Here's how the part is built. I have some questions about the finished solid (model axes, mm). Round coordinates to 2 decimals unless told otherwise and drop trailing zeros. Order: outer loops, then holes, each group sorted by start corner. A loop starts at its lowest first (then second) coordinate and runs counter-clockwise, first axis right, second up. Notation, with made-up numbers: (73, 21.25) - (78, 21.25) arc R28 cw to (78, 54.25) - close; hole circle Ø8 at (15.25, -1). An arc over 180 degrees is marked (long way). Answer as a JSON object with one key per item and string values.
```python
from build123d import *

# Parameters (mm, degrees)
SKETCH1_W           = 12.7
SKETCH1_H           = 25.4
SKETCH1_W_2         = 9.525
SKETCH1_H_2         = 22.225
BOSS_EXTRUDE1_DEPTH = 609.6
SKETCH2_R           = 3.81
SKETCH2_R_2         = 2.75
CUT_EXTRUDE1_DEPTH  = 610.86452594
CUT_EXTRUDE3_REACH  = 611.865
CUT_EXTRUDE5_REACH  = 612.162
SKETCH5_R           = 2.75


with BuildPart() as part:
    # Sketch1 → Boss-Extrude1 (new body)
    with BuildSketch(Plane.XY):
        Rectangle(SKETCH1_W, SKETCH1_H)
        Rectangle(SKETCH1_W_2, SKETCH1_H_2, mode=Mode.SUBTRACT)
    extrude(amount=BOSS_EXTRUDE1_DEPTH)

    # Sketch2 → Cut-Extrude1 (cut, through all)
    with BuildSketch(Plane(origin=(6.35, 0, 0), x_dir=(0, 0, -1), z_dir=(1, 0, 0))):
        with Locations((-571.5, 0)):
            Circle(SKETCH2_R)
        with Locations((-586.74, 0)):
            Circle(SKETCH2_R_2)
        with Locations((-556.26, 0)):
            Circle(SKETCH2_R_2)
        with Locations((-66.04, 0)):
            Circle(SKETCH2_R_2)
        with Locations((-35.56, 0)):
            Circle(SKETCH2_R_2)
        with Locations((-382.778, 0)):
            Circle(SKETCH2_R_2)
        with Locations((-398.018, 0)):
            Circle(SKETCH2_R)
        with Locations((-413.258, 0)):
            Circle(SKETCH2_R_2)
        with Locations((-209.296, 0)):
            Circle(SKETCH2_R_2)
        with Locations((-224.536, 0)):
            Circle(SKETCH2_R)
        with Locations((-239.776, 0)):
            Circle(SKETCH2_R_2)
        with BuildLine():
            Line((-44.45, -3.302), (-57.15, -3.302))
            ThreePointArc((-57.15, -3.302), (-60.452, 0), (-57.15, 3.302))
            Line((-57.15, 3.302), (-44.45, 3.302))
            ThreePointArc((-44.45, 3.302), (-41.148, 0), (-44.45, -3.302))
        make_face()
    extrude(amount=-CUT_EXTRUDE1_DEPTH, mode=Mode.SUBTRACT)

    # Sketch4 → Cut-Extrude3 (cut, up to next)
    with BuildSketch(Plane.ZY.offset(6.35), mode=Mode.PRIVATE) as cut_extrude3_sk1:
        with BuildLine():
            Line((35.56, 5), (66.04, 5))
            ThreePointArc((66.04, 5), (71.04, 0), (66.04, -5))
            Line((66.04, -5), (35.56, -5))
            ThreePointArc((35.56, -5), (30.56, 0), (35.56, 5))
        make_face()
    cut_extrude3_tool1 = extrude(cut_extrude3_sk1.sketch, amount=-CUT_EXTRUDE3_REACH, mode=Mode.PRIVATE) & part.part
    # Sketch4 → Cut-Extrude3 (cut, up to next)
    with BuildSketch(Plane.ZY.offset(6.35), mode=Mode.PRIVATE) as cut_extrude3_sk2:
        with BuildLine():
            Line((556.26, 5), (586.74, 5))
            ThreePointArc((586.74, 5), (591.74, 0), (586.74, -5))
            Line((586.74, -5), (556.26, -5))
            ThreePointArc((556.26, -5), (551.26, 0), (556.26, 5))
        make_face()
    cut_extrude3_tool2 = extrude(cut_extrude3_sk2.sketch, amount=-CUT_EXTRUDE3_REACH, mode=Mode.PRIVATE) & part.part
    # Sketch4 → Cut-Extrude3 (cut, up to next)
    with BuildSketch(Plane.ZY.offset(6.35), mode=Mode.PRIVATE) as cut_extrude3_sk3:
        with BuildLine():
            Line((209.042, 5), (239.522, 5))
            ThreePointArc((239.522, 5), (244.522, 0), (239.522, -5))
            Line((239.522, -5), (209.042, -5))
            ThreePointArc((209.042, -5), (204.042, 0), (209.042, 5))
        make_face()
    cut_extrude3_tool3 = extrude(cut_extrude3_sk3.sketch, amount=-CUT_EXTRUDE3_REACH, mode=Mode.PRIVATE) & part.part
    # Sketch4 → Cut-Extrude3 (cut, up to next)
    with BuildSketch(Plane.ZY.offset(6.35), mode=Mode.PRIVATE) as cut_extrude3_sk4:
        with BuildLine():
            Line((382.524, 5), (413.004, 5))
            ThreePointArc((413.004, 5), (418.004, 0), (413.004, -5))
            Line((413.004, -5), (382.524, -5))
            ThreePointArc((382.524, -5), (377.524, 0), (382.524, 5))
        make_face()
    cut_extrude3_tool4 = extrude(cut_extrude3_sk4.sketch, amount=-CUT_EXTRUDE3_REACH, mode=Mode.PRIVATE) & part.part
    add(cut_extrude3_tool1.solids().sort_by_distance((-6.35, 0, 50.8))[0], mode=Mode.SUBTRACT)
    add(cut_extrude3_tool2.solids().sort_by_distance((-6.35, 0, 571.5))[0], mode=Mode.SUBTRACT)
    add(cut_extrude3_tool3.solids().sort_by_distance((-6.35, 0, 224.282))[0], mode=Mode.SUBTRACT)
    add(cut_extrude3_tool4.solids().sort_by_distance((-6.35, 0, 397.764))[0], mode=Mode.SUBTRACT)

    # Sketch5 → Cut-Extrude5 (cut, up to next)
    with BuildSketch(Plane.XZ.offset(12.7), mode=Mode.PRIVATE) as cut_extrude5_sk1:
        with Locations(Location((0, 596.9, 0), (0, 0, 270))):
            Circle(SKETCH5_R)
    cut_extrude5_tool1 = extrude(cut_extrude5_sk1.sketch, amount=-CUT_EXTRUDE5_REACH, mode=Mode.PRIVATE) & part.part
    # Sketch5 → Cut-Extrude5 (cut, up to next)
    with BuildSketch(Plane.XZ.offset(12.7), mode=Mode.PRIVATE) as cut_extrude5_sk2:
        with Locations(Location((0, 12.7, 0), (0, 0, 270))):
            Circle(SKETCH5_R)
    cut_extrude5_tool2 = extrude(cut_extrude5_sk2.sketch, amount=-CUT_EXTRUDE5_REACH, mode=Mode.PRIVATE) & part.part
    add(cut_extrude5_tool1.solids().sort_by_distance((0, -12.7, 596.9))[0], mode=Mode.SUBTRACT)
    add(cut_extrude5_tool2.solids().sort_by_distance((0, -12.7, 12.7))[0], mode=Mode.SUBTRACT)


solid = part.part
```
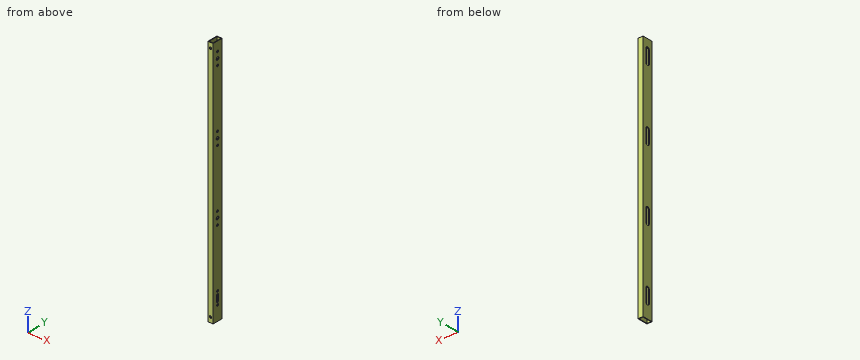
1. For P1, Ø5, axis at y = 0, z = 209.296, coming from the +X side, with a flat end and sliding along its axis, tell me the tip position at first contact or that it passes through.
Responses:
{"P1": "through"}
2. Imagine slicing it at B-B (z = 291). List the corners of the cut face in (x, y) for me.
Responses:
{"outline": "(-6.35, -12.7) - (6.35, -12.7) - (6.35, 12.7) - (-6.35, 12.7) - close; hole (-4.76, -11.11) - (4.76, -11.11) - (4.76, 11.11) - (-4.76, 11.11) - close"}
3. If I drill on L1, parallel to Y at x = 0.75, z = 227; L2, parallel to X at y = 10.5, z = 569.5; L3, parallel to Y at x = 5.6, z = 35.56, over which ranges is the centre line in solid material (lowest first)? Write a range as [from, to].
Responses:
{"L1": "[-12.7, -11.11], [11.11, 12.7]", "L2": "[-6.35, -4.76], [4.76, 6.35]", "L3": "[-12.7, -2.75], [2.75, 12.7]"}
4. Imagine slicing it at A-A (x = 0). List the corners of the cut face in (y, z) for me, plus the area to 3 significant figures.
Responses:
{"outline": "(-12.7, 0) - (-11.11, 0) - (-11.11, 9.95) - (-12.7, 9.95) - close; (-12.7, 15.45) - (-11.11, 15.45) - (-11.11, 594.15) - (-12.7, 594.15) - close; (-12.7, 599.65) - (-11.11, 599.65) - (-11.11, 609.6) - (-12.7, 609.6) - close; (11.11, 0) - (12.7, 0) - (12.7, 609.6) - (11.11, 609.6) - close", "area": "1,920 mm2"}
